from build123d import *

# Parameters (mm, degrees)
SKETCH3_R                                            = 60.625
SKETCH3_R_2                                          = 45
BOSS_EXTRUDE1_DEPTH                                  = 4
SKETCH5_R                                            = 49
SKETCH5_R_2                                          = 45
BOSS_EXTRUDE2_DEPTH                                  = 52
SKETCH6_W                                            = 8
SKETCH6_H                                            = 38
BOSS_EXTRUDE3_DEPTH                                  = 13
SKETCH7_W                                            = 10
SKETCH7_H                                            = 24
CUT_EXTRUDE1_DEPTH                                   = 26
SKETCH8_R                                            = 5
CUT_EXTRUDE2_DEPTH                                   = 55
SKETCH9_R                                            = 1.3
CUT_EXTRUDE5_DEPTH                                   = 7.2
BOSS_EXTRUDE5_DEPTH                                  = 4
CSK_FOR_ST2_2_CROSS_RECESSED_CTSK_HEAD_T_D           = 2.6
CSK_FOR_ST2_2_CROSS_RECESSED_CTSK_HEAD_T_CSINK_D     = 4.4
CSK_FOR_ST2_2_CROSS_RECESSED_CTSK_HEAD_T_CSINK_ANGLE = 90
FILLET1_R                                            = 1


with BuildPart() as part:
    # Sketch3 → Boss-Extrude1 (new body)
    with BuildSketch(Plane(origin=(0, 0, 0), x_dir=(1, 0, 0), z_dir=(0, 1, 0))):
        with Locations(Location((0, 0, 0), (0, 0, 270))):
            Circle(SKETCH3_R)
        with Locations(Location((0, 0, 0), (0, 0, 270))):
            Circle(SKETCH3_R_2, mode=Mode.SUBTRACT)
    extrude(amount=BOSS_EXTRUDE1_DEPTH)

    # Sketch5 → Boss-Extrude2 (add)
    with BuildSketch(Plane(origin=(0, 4, 0), x_dir=(1, 0, 0), z_dir=(0, 1, 0))):
        with Locations(Location((0, 0, 0), (0, 0, 90))):
            Circle(SKETCH5_R)
        with Locations(Location((0, 0, 0), (0, 0, 270))):
            Circle(SKETCH5_R_2, mode=Mode.SUBTRACT)
    extrude(amount=BOSS_EXTRUDE2_DEPTH)

    # Sketch6 → Boss-Extrude3 (add, symmetric)
    with BuildSketch(Plane(origin=(0, 0, 0), x_dir=(0, 0, -1), z_dir=(1, 0, 0))):
        Polygon((-46.75, 38), (-31.75, 38), (-31.75, 30), (-45, 16.75), (-46.75, 15), (-46.75, 30), align=None)
        with Locations((15.25, 19)):
            Rectangle(SKETCH6_W, SKETCH6_H)
    extrude(amount=BOSS_EXTRUDE3_DEPTH, both=True)


with BuildPart() as boss_extrude3_piece_1:
    # of the separate pieces the step leaves, piece 1, a body of its own (boss_extrude3_pieces)
    add(part.part.solids().sort_by_distance((0, 0, 60.625))[0])

    # Sketch8 → Cut-Extrude2 (cut)
    with BuildSketch(Plane.XY.offset(-11.25)):
        with Locations(Location((0, 14, 0), (0, 0, 90))):
            Circle(SKETCH8_R)
    extrude(amount=-CUT_EXTRUDE2_DEPTH, mode=Mode.SUBTRACT)


with BuildPart() as boss_extrude3_piece_2:
    # of the separate pieces the step leaves, piece 2, a body of its own (boss_extrude3_pieces)
    add(part.part.solids().sort_by_distance((-13, 38, -11.25))[0])

    # Sketch7 → Cut-Extrude1 (cut)
    with BuildSketch(Plane.XY.offset(-11.25)):
        with Locations((0, 17)):
            Rectangle(SKETCH7_W, SKETCH7_H)
    extrude(amount=-CUT_EXTRUDE1_DEPTH, mode=Mode.SUBTRACT)


with BuildPart() as cut_extrude5_tool:
    # Sketch9 → Cut-Extrude5 (new body)
    with BuildSketch(Plane(origin=(0, 38, 0), x_dir=(1, 0, 0), z_dir=(0, 1, 0))):
        with Locations(Location((5, 13.75, 0), (0, 0, 270))):
            Circle(SKETCH9_R)
        with Locations(Location((5, -34.25, 0), (0, 0, 270))):
            Circle(SKETCH9_R)
        with Locations(Location((-5, -34.25, 0), (0, 0, 270))):
            Circle(SKETCH9_R)
        with Locations(Location((-5, 13.75, 0), (0, 0, 270))):
            Circle(SKETCH9_R)
    extrude(amount=-CUT_EXTRUDE5_DEPTH)


with BuildPart() as boss_extrude3_piece_1_1:
    add(boss_extrude3_piece_1.part)

    # Cut-Extrude5: cut by cut_extrude5_tool
    add(cut_extrude5_tool.part, mode=Mode.SUBTRACT)



with BuildPart() as boss_extrude3_piece_2_1:
    add(boss_extrude3_piece_2.part)

    # Cut-Extrude5: cut by cut_extrude5_tool
    add(cut_extrude5_tool.part, mode=Mode.SUBTRACT)


with BuildPart() as boss_extrude3_piece_1_2:
    add(boss_extrude3_piece_1_1.part)

    add(boss_extrude3_piece_2_1.part)  # Boss-Extrude5 merges Boss-Extrude3 piece 2
    # Sketch10 → Boss-Extrude5 (add)
    with BuildSketch(Plane.XZ):
        with BuildLine():
            Line((37.248431585, -25.249838503), (13, -11.25))
            Line((13, -11.25), (-13, -11.25))
            Line((-13, -11.25), (-37.248431585, -25.249838503))
            ThreePointArc((-37.248431585, -25.249838503), (0, -45), (37.248431585, -25.249838503))
        make_face()
        with BuildLine():
            Line((-19.516660498, -24.25), (19.516660498, -24.25))
            Line((19.516660498, -24.25), (24.906460381, -27.361802413))
            ThreePointArc((24.906460381, -27.361802413), (0, -37), (-24.906460381, -27.361802413))
            Line((-24.906460381, -27.361802413), (-19.516660498, -24.25))
        make_face(mode=Mode.SUBTRACT)
    extrude(amount=-BOSS_EXTRUDE5_DEPTH)

    # CSK for ST2.2 Cross recessed CTSK head tapping screws1 (through all)
    with Locations(Plane(origin=(0, 4, 0), x_dir=(1, 0, 0), z_dir=(0, 1, 0))):
        with Locations((0, 0), (38, -40), (-38, 40), (-38, -40), (38, 40)):
            CounterSinkHole(CSK_FOR_ST2_2_CROSS_RECESSED_CTSK_HEAD_T_D / 2, CSK_FOR_ST2_2_CROSS_RECESSED_CTSK_HEAD_T_CSINK_D / 2, counter_sink_angle=CSK_FOR_ST2_2_CROSS_RECESSED_CTSK_HEAD_T_CSINK_ANGLE)

    # Fillet1
    fillet1_edges = [boss_extrude3_piece_1_2.edges().sort_by_distance(p)[0] for p in [
        (0, 4, 49),
    ]]
    fillet(fillet1_edges, radius=FILLET1_R)


solid = boss_extrude3_piece_1_2.part
Verification items for the finished model (mm, model axes). A direction names the side the tool comes from. Coordinates: 2 decimals unless noted, no trailing zeros. Loops run counter-clockwise (first coordinate to the right, second up) from the corner with the lowest first, then second, coordinate; pieces in that order, holes last. Notation, with made-up numbers: (0.25, 55.25) -> (44.25, 55.25) arc R35 cw to (44.25, 91.25) -> close; hole circle Ø6 at (58, 50.5). An arc over 180 degrees is marked (long way). Write each question's results on one line, items separated by ' | '.
Item 1: Gauge pin test, flat ends, axial feed: pin 1 (2.5 mm diameter, centred on x = -5, z = -13.75, fed in from -Y); pin 2 (6 mm diameter, centred on x = -22, y = 45, fed in from +Z); pin 3 (4 mm diameter, centred on x = 25.5, y = 46.5, fed in from -Z); pin 4 (2 mm diameter, centred on y = 28, z = 26.5, fed in from -X). Record the tip position at first contact, or that the pin passes through.
Found:
pin 1: stops at y = 0 | pin 2: stops at z = 45.17 | pin 3: stops at z = -43 | pin 4: stops at x = -41.84
Item 2: Mould release check, pull along Z, two halves, no side actions. Record for faces 1 (the face through (5, 17, -15)), 2 (the face through (13, 21, -15)), 3 (the face through (22, 56, -40)): +Z half, -Z half, draft (parallel to the pull), parting line (faces both ways), or undercut.
Found:
face 1: undercut | face 2: undercut | face 3: draft
Item 3: Section check C-C, the plane y = 15. Enter the section's corners in (x, z), plus the area to 3 significant figures.
Found:
outline: (-13, -19.25) -> (-5, -19.25) -> (-5, -11.25) -> (-13, -11.25) -> close; (-4.9, -48.75) -> (-4.9, -44.73) arc R45 cw (long way) to (4.9, -44.73) -> (4.9, -48.75) arc R49 ccw (long way) to start; (5, -19.25) -> (13, -19.25) -> (13, -11.25) -> (5, -11.25) -> close | area: 1,270 mm2
Item 4: Section check B-B, the plane x = 0. Count the separate pieces of the cut face and the enclosed holes in it, plus the area to 3 significant figures.
Found:
separate pieces: 5 | enclosed holes: 0 | area: 859 mm2
Item 5: Section check A-A, the plane z = 0. Enter the section's corners in (x, y) (3 decimals), plus the area to 3 significant figures.
Found:
outline: (-60.625, 0) -> (-45, 0) -> (-45, 56) -> (-49, 56) -> (-49, 5) arc R1 cw to (-50, 4) -> (-60.625, 4) -> close; (45, 0) -> (60.625, 0) -> (60.625, 4) -> (50, 4) arc R1 cw to (49, 5) -> (49, 56) -> (45, 56) -> close | area: 541 mm2
Item 6: Tool access check on faces 4 (the face through (0, 29, -15)), 5 (the face through (0, 2, -24.25)), 6 (the face through (0, 38, -15)). Record the directions out of +Z, -Z, +X, -X, +Y, -Y that give a thin tool (end or side, any length) a straight path to the whole face; none if there is none.
Found:
face 4: none | face 5: +Y, -Y | face 6: +Y
Item 7: Material ranges on L1, parallel to X at y = 22, z = 0; L2, parallel to Z at x = -10.5, y = 29; L3, parallel to X at y = 35.75, z = -13.75, recorded low to high.
Found:
L1: x = -49 to -45, 45 to 49 | L2: z = -47.86 to -43.76, -19.25 to -11.25, 32.75 to 47.86 | L3: x = -47.03 to -42.85, -13 to -6.3, -3.7 to 3.7, 6.3 to 13, 42.85 to 47.03
